Read the model definition and answer for the solid it produces. Units are mm, in the model's axes. Face numbers are marked on the shaded views. Coordinates: 2 decimals unless noted, no trailing zeros. Order: outer loops, then holes, each group sorted by start corner. A loop starts at its lowest first (then second) coordinate and runs counter-clockwise, first axis right, second up. Notation, with made-up numbers: (3, 89) -> (53, 89) arc R34 ccw to (53, 120) -> close; hole circle Ø10 at (-14, 21). An arc over 180 degrees is marked (long way). Answer in a Markdown table with one row per item.
from build123d import *

# Parameters (mm, degrees)
F2_R = 1
F3_R = 0.99999


# Not quite as in the source:
# - a fillet or chamfer is up to 0.001 mm smaller than in the source, because OpenCascade refuses the exact size


with BuildPart() as f1:
    # F0 (on Front) → F1 (revolve)
    with BuildSketch(Plane.XZ):
        with BuildLine():
            Line((0, 0), (35, 0))
            Line((35, 0), (35, 2))
            Line((35, 2), (14.6711988598, 2))
            ThreePointArc((14.6711988598, 2), (6.4184150015, 5.4184150015), (3, 13.6711988598))
            Line((3, 13.6711988598), (3, 60))
            ThreePointArc((3, 60), (5.2663701885, 73.0449457567), (11.7998654023, 84.5610424876))
            Line((11.7998654023, 84.5610424876), (30.1194867973, 106.8448902178))
            ThreePointArc((30.1194867973, 106.8448902178), (35.9954931852, 118.4070626292), (36.4419899072, 131.3690039428))
            Line((36.4419899072, 131.3690039428), (25.5640022925, 190))
            Line((25.5640022925, 190), (24.5469366539, 190))
            Line((24.5469366539, 190), (24.716161279, 189.0879003841))
            Line((24.716161279, 189.0879003841), (35.4587691965, 131.186584004))
            ThreePointArc((35.4587691965, 131.186584004), (35.0271556985, 118.6567074008), (29.3470161902, 107.4799407364))
            Line((29.3470161902, 107.4799407364), (11.0273947953, 85.1960930063))
            ThreePointArc((11.0273947953, 85.1960930063), (4.3249694749, 73.3822359826), (2, 60))
            Line((2, 60), (0, 60))
            Line((0, 60), (0, 0))
        make_face()
    revolve(axis=Axis((0, 0, -18.4489581734), (0, 0, -1)))

    # F2
    f2_edges = [f1.edges().sort_by_distance(p)[0] for p in [
        (-35, 0, 2),
    ]]
    fillet(f2_edges, radius=F2_R)

    # F3 (radius 1 in the source; OpenCascade refuses exactly that, so slightly less here)
    f3_edges = [f1.edges().sort_by_distance(p)[0] for p in [
        (-35, 0, 0),
    ]]
    fillet(f3_edges, radius=F3_R)


solid = f1.part
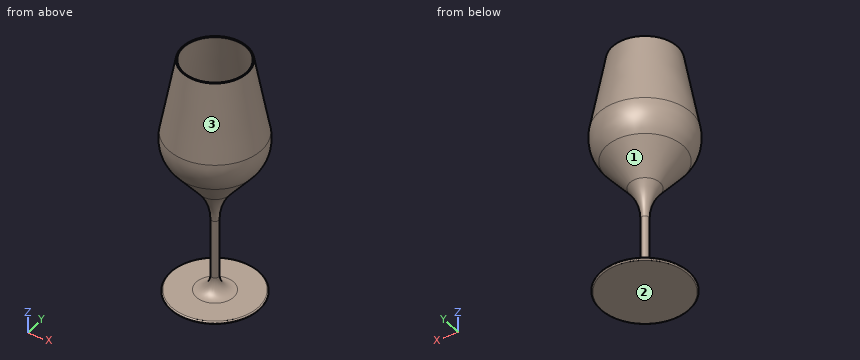
Q1. For a pull along Z with two mould halves and no side action, classify the marked faces 1, 2 and 3 as pulls with the +Z half, pulls with the -Z half, needs draft (parallel to the pull), parting line crosses it, or undercut.
Outcome:
| item | result |
|---|---|
| face 1 | undercut |
| face 2 | pulls with the -Z half |
| face 3 | pulls with the +Z half |
Q2. Consider line 1 (Y direction, x = -10, z = 140.5); line 2 (X direction, y = -22, z = 147.5); line 3 (Y direction, x = 9, z = 181). Determine where each line is inside the solid, lowest interval first.
Outcome:
| item | result |
|---|---|
| line 1 | -33.28 to -32.21, 32.21 to 33.28 |
| line 2 | -25.2 to -23.83, 23.83 to 25.2 |
| line 3 | -25.7 to -24.62, 24.62 to 25.7 |
Q3. The part is cut by section C-C (z = 92). Write down the section's boundary in (x, y).
Outcome:
| item | result |
|---|---|
| outline | circle Ø35.83 at (0, 0); hole circle Ø33.24 at (0, 0) |
Q4. Given pin 1 (3 mm diameter, centred on x = 12, z = 103.5, fed in from -Y); pin 2 (1.2 mm diameter, centred on x = 1, y = 0.5, fed in from +Z); pin 3 (1 mm diameter, centred on y = 27, z = 163.5, fed in from -X); pin 4 (10 mm diameter, centred on y = 11, z = 42, fed in from -X), each flat-ended and moving along its own axis, determine where each tip first touches the part or whether it passes through.
Outcome:
| item | result |
|---|---|
| pin 1 | y = -26.12 |
| pin 2 | z = 60 |
| pin 3 | x = -15.08 |
| pin 4 | through |
Q5. The part is cut by section A-A (y = -32). Give the number of separate pieces and of enclosed holes in the cut face, then the cut area to 3 significant figures.
Outcome:
| item | result |
|---|---|
| separate pieces | 2 |
| enclosed holes | 1 |
| area | 360 mm² |
Q6. The part is cut by section B-B (z = 57). Write down the section's boundary in (x, y).
Outcome:
| item | result |
|---|---|
| outline | circle Ø6 at (0, 0) |
